Geometry check sheet. Reference: the model listing, model coordinates, mm. Face numbers are marked on the shaded views. Coordinates: 2 decimals unless noted, no trailing zeros. Order: outer loops, then holes, each group sorted by start corner. A loop starts at its lowest first (then second) coordinate and runs counter-clockwise, first axis right, second up.
```python
from build123d import *

# Parameters (mm, degrees)
SKETCH036_R       = 1.6
PAD001_DEPTH      = 61.5
PAD001_DEPTH_BACK = 61.5
SKETCH037_W       = 16.5
SKETCH037_H       = 8
POCKET_DEPTH      = 4
POCKET_DEPTH_BACK = 4
SKETCH044_W       = 119
SKETCH044_H       = 67.4
POCKET007_DEPTH   = 2
SKETCH045_W       = 114.6
SKETCH045_H       = 63
POCKET008_DEPTH   = 9
SKETCH046_R       = 1.8
PAD002_DEPTH      = 9
SKETCH047_W       = 56.5
SKETCH047_H       = 30.7
POCKET009_DEPTH   = 7.8
SKETCH048_R       = 1.2
POCKET010_DEPTH   = 2
SKETCH052_W       = 16.5
SKETCH052_H       = 4
POCKET014_DEPTH   = 0.4
SKETCH053_W       = 14.4
SKETCH053_H       = 5.5
POCKET015_DEPTH   = 2.2
SKETCH054_W       = 14
SKETCH054_H       = 6
POCKET016_DEPTH   = 2
SKETCH055_R       = 3
POCKET017_DEPTH   = 4
SKETCH056_R       = 3
POCKET018_DEPTH   = 4


with BuildPart() as part:
    # Sketch036 (on Face1 of Binder001) → Pad001 (new body, two sides)
    with BuildSketch(Plane.YZ) as pad001_sk:
        with BuildLine():
            ThreePointArc((0, -4), (2.828427, 2.828427), (-4, 0))
            Line((-75.8, 0), (-4, 0))
            Line((-75.8, -13), (-75.8, 0))
            Line((-4.4, -13), (-75.8, -13))
            Line((-4.4, -4), (-4.4, -13))
            Line((0, -4), (-4.4, -4))
        make_face()
        Circle(SKETCH036_R, mode=Mode.SUBTRACT)
    extrude(amount=PAD001_DEPTH)
    extrude(pad001_sk.sketch, amount=-PAD001_DEPTH_BACK)

    # Sketch037 → Pocket (cut, two sides)
    with BuildSketch(Plane.XY) as pocket_sk:
        with Locations((-38.25, 0)):
            Rectangle(SKETCH037_W, SKETCH037_H)
        with Locations((38.25, 0)):
            Rectangle(SKETCH037_W, SKETCH037_H)
    extrude(amount=-POCKET_DEPTH, mode=Mode.SUBTRACT)
    extrude(pocket_sk.sketch, amount=POCKET_DEPTH_BACK, mode=Mode.SUBTRACT)

    # Sketch044 → Pocket007 (cut)
    with BuildSketch(Plane.XY):
        with Locations((0, -40.1)):
            Rectangle(SKETCH044_W, SKETCH044_H)
    extrude(amount=-POCKET007_DEPTH, mode=Mode.SUBTRACT)

    # Sketch045 (on Face23 of Pocket007) → Pocket008 (cut)
    with BuildSketch(Plane.XY.offset(-2)):
        with Locations((0, -40.1)):
            Rectangle(SKETCH045_W, SKETCH045_H)
    extrude(amount=-POCKET008_DEPTH, mode=Mode.SUBTRACT)

    # Sketch046 (on Face29 of Pocket008) → Pad002 (join)
    with BuildSketch(Plane.XY.offset(-11)):
        with BuildLine():
            ThreePointArc((-54.3, -43.1), (-51.3, -40.1), (-54.3, -37.1))
            Line((-57.3, -37.1), (-54.3, -37.1))
            Line((-57.3, -43.1), (-57.3, -37.1))
            Line((-54.3, -43.1), (-57.3, -43.1))
        make_face()
        with Locations((-54.3, -40.1)):
            Circle(SKETCH046_R, mode=Mode.SUBTRACT)
        with BuildLine():
            ThreePointArc((-3, -11.6), (0, -14.6), (3, -11.6))
            Line((3, -8.6), (3, -11.6))
            Line((-3, -8.6), (3, -8.6))
            Line((-3, -11.6), (-3, -8.6))
        make_face()
        with Locations((0, -11.6)):
            Circle(SKETCH046_R, mode=Mode.SUBTRACT)
        with BuildLine():
            ThreePointArc((54.3, -37.1), (51.3, -40.1), (54.3, -43.1))
            Line((57.3, -43.1), (54.3, -43.1))
            Line((57.3, -37.1), (57.3, -43.1))
            Line((54.3, -37.1), (57.3, -37.1))
        make_face()
        with Locations((54.3, -40.1)):
            Circle(SKETCH046_R, mode=Mode.SUBTRACT)
        with BuildLine():
            ThreePointArc((3, -68.6), (0, -65.6), (-3, -68.6))
            Line((-3, -68.6), (-3, -71.6))
            Line((-3, -71.6), (3, -71.6))
            Line((3, -71.6), (3, -68.6))
        make_face()
        with Locations((0, -68.6)):
            Circle(SKETCH046_R, mode=Mode.SUBTRACT)
    extrude(amount=PAD002_DEPTH)

    # Sketch047 (on Face24 of Pad002) → Pocket009 (cut)
    with BuildSketch(Plane.XY.offset(-2)):
        with Locations((-31.25, -21.75)):
            Rectangle(SKETCH047_W, SKETCH047_H)
        with Locations((31.25, -21.75)):
            Rectangle(SKETCH047_W, SKETCH047_H)
        with Locations((31.25, -58.45)):
            Rectangle(SKETCH047_W, SKETCH047_H)
        with Locations((-31.25, -58.45)):
            Rectangle(SKETCH047_W, SKETCH047_H)
    extrude(amount=-POCKET009_DEPTH, mode=Mode.SUBTRACT)

    # Sketch048 (on Face6 of Pocket009) → Pocket010 (cut)
    with BuildSketch(Plane.XZ.offset(75.8)):
        with Locations((-5, -6.4)):
            Circle(SKETCH048_R)
        with Locations((5, -6.4)):
            Circle(SKETCH048_R)
    extrude(amount=-POCKET010_DEPTH, mode=Mode.SUBTRACT)

    # Sketch052 (on Face13 of Pocket010) → Pocket014 (cut)
    with BuildSketch(Plane(origin=(0, -4, 0), x_dir=(-1, 0, 0), z_dir=(0, 1, 0))):
        with Locations((38.25, -2)):
            Rectangle(SKETCH052_W, SKETCH052_H)
        with Locations((-38.25, -2)):
            Rectangle(SKETCH052_W, SKETCH052_H)
    extrude(amount=-POCKET014_DEPTH, mode=Mode.SUBTRACT)

    # Sketch053 (on Face58 of Pocket014) → Pocket015 (cut)
    with BuildSketch(Plane(origin=(0, -4.4, 0), x_dir=(-1, 0, 0), z_dir=(0, 1, 0))):
        with Locations((-28.1, -5.05)):
            Rectangle(SKETCH053_W, SKETCH053_H)
    extrude(amount=-POCKET015_DEPTH, mode=Mode.SUBTRACT)

    # Sketch054 (on Face15 of Pocket015) → Pocket016 (cut)
    with BuildSketch(Plane.YZ.offset(61.5)):
        with Locations((-59.2, -5)):
            Rectangle(SKETCH054_W, SKETCH054_H)
    extrude(amount=-POCKET016_DEPTH, mode=Mode.SUBTRACT)

    # Sketch055 (on Face15 of Pocket016) → Pocket017 (cut)
    with BuildSketch(Plane.YZ.offset(61.5)):
        Circle(SKETCH055_R)
    extrude(amount=-POCKET017_DEPTH, mode=Mode.SUBTRACT)

    # Sketch056 (on Face2 of Pocket017) → Pocket018 (cut)
    with BuildSketch(Plane(origin=(-61.5, 0, 0), x_dir=(0, -1, 0), z_dir=(-1, 0, 0))):
        Circle(SKETCH056_R)
    extrude(amount=-POCKET018_DEPTH, mode=Mode.SUBTRACT)


solid = part.part
```
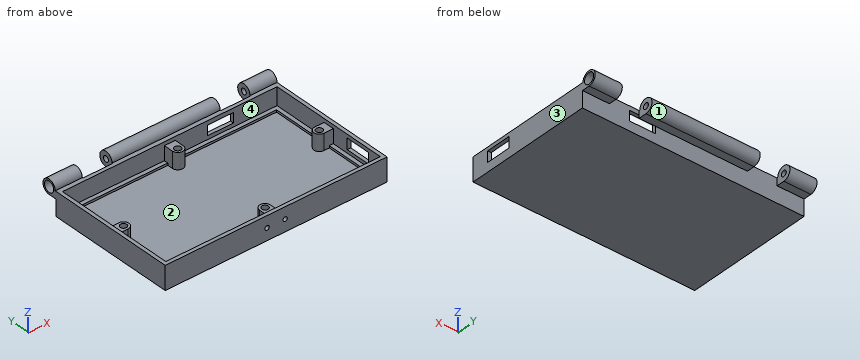
Item 1: Sectioned sample at D-D (y = -22.5). Record the cut outline in (x, z).
Item 2: Sectioned sample at B-B (y = -54.5). Record the cut outline in (x, z), and give its area (3 significant figures).
Item 3: Release check for a two-part mould opening along Y. For the marked faces 1, 2, 3 and 4 record: pulls with the +Y half, pulls with the -Y half, needs draft (parallel to the pull), parting line crosses it, or undercut.
Item 4: Sectioned sample at C-C (x = -25). Record the cut outline in (y, z), and give its area (3 significant figures).
Item 5: Thickness scan on line 1 along X through (y, z) = (-1, 3); line 2 along X through (y, z) = (-22, -8.75); line 3 along X through (y, z) = (-1, -2). Record the ranges inside material, lowest first.
Item 6: Sectioned sample at A-A (x = 5). Record the cut outline in (y, z).
Item 7: Depth check by flat-ended pin: P1, Ø2.5, axis at y = 0, z = -0.5, coming from the +X side; P2, Ø1.5, axis at x = -43.5, y = -44, coming from the +Z side; P3, Ø0.6, axis at x = 27.5, z = -10.5, coming from the +Y side. Enter the tip coordinate at first touch or a pass-through.
Geometry check:
1. outline: (-61.5, -13) - (61.5, -13) - (61.5, 0) - (59.5, 0) - (59.5, -9.8) - (57.3, -9.8) - (57.3, -11) - (-57.3, -11) - (-57.3, -9.8) - (-59.5, -9.8) - (-59.5, 0) - (-61.5, 0) - close
2. outline: (-61.5, -13) - (61.5, -13) - (61.5, -8) - (59.5, -8) - (59.5, -9.8) - (57.3, -9.8) - (57.3, -11) - (-57.3, -11) - (-57.3, -9.8) - (-59.5, -9.8) - (-59.5, 0) - (-61.5, 0) - close; (59.5, -2) - (61.5, -2) - (61.5, 0) - (59.5, 0) - close
2. area: 283 mm2
3. face 1: parting line crosses it
3. face 2: undercut
3. face 3: needs draft
3. face 4: undercut
4. outline: (-75.8, -13) - (-4.4, -13) - (-4.4, -4) - (0, -4) arc R4 ccw (long way) to (-4, 0) - (-6.4, 0) - (-6.4, -9.8) - (-8.6, -9.8) - (-8.6, -11) - (-71.6, -11) - (-71.6, -9.8) - (-73.8, -9.8) - (-73.8, 0) - (-75.8, 0) - close; hole circle Ø3.2 at (0, 0)
4. area: 239 mm2
5. line 1: x = -61.5 to -46.5, -30 to 30, 46.5 to 61.5
5. line 2: x = -61.5 to -59.5, 59.5 to 61.5
5. line 3: x = -57.5 to -46.5, -30 to 30, 46.5 to 57.5
6. outline: (-75.8, -13) - (-4.4, -13) - (-4.4, -4) - (0, -4) arc R4 ccw (long way) to (-4, 0) - (-6.4, 0) - (-6.4, -9.8) - (-8.6, -9.8) - (-8.6, -11) - (-71.6, -11) - (-71.6, -9.8) - (-73.8, -9.8) - (-73.8, -7.6) - (-75.8, -7.6) - close; (-75.8, -5.2) - (-73.8, -5.2) - (-73.8, 0) - (-75.8, 0) - close; hole circle Ø3.2 at (0, 0)
7. P1: stops at x = 57.5
7. P2: stops at z = -11
7. P3: stops at y = -4.4
